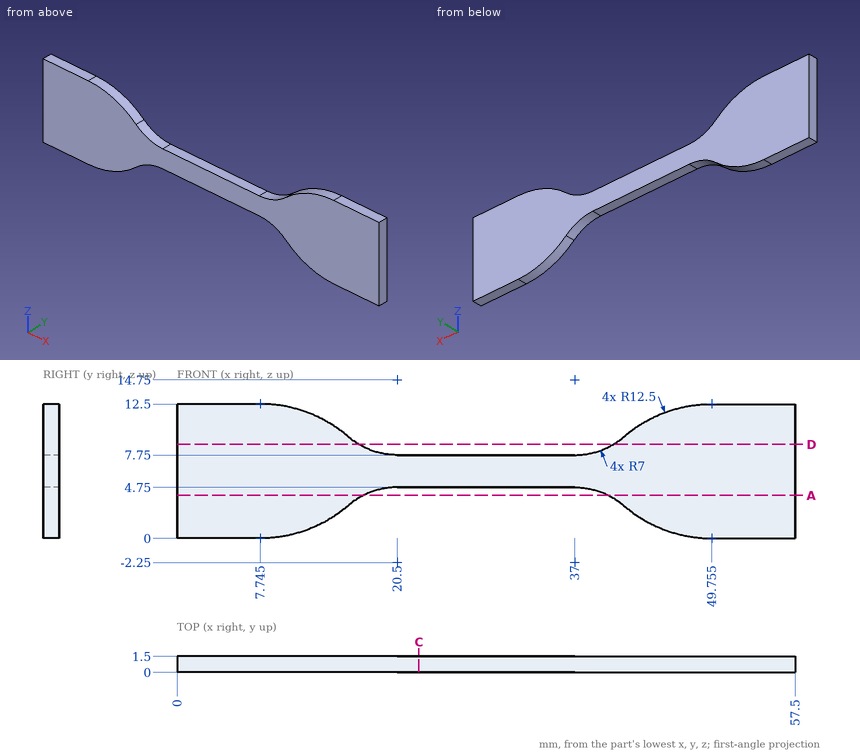
Source: three-view drawing plus pictorial views. Frame: mm from the lowest corner of the part. Give positions to 0.01 mm unless a question says otherwise; leave off trailing zeros. Order: outer loops, then holes, each group sorted by start corner. A loop starts at its lowest first (then second) coordinate and runs counter-clockwise, first axis right, second up. Notation, with made-up numbers: (17.25, 54) - (47.25, 54) arc R16 cw to (47.25, 65) - close; hole circle Ø7 at (1.5, 46.25). An arc over 180 degrees is marked (long way). Answer as a JSON object with one key per item and string values. Group by question number.
Q1. Cut plane C-C, the plane x = 22.5. Output: boundary loops of the cut face in (y, z).
Q2. Line query: probe 1 along Z at (x, y) = (8, 0.75); probe 2 along X at (y, z) = (1, 3.25); probe 3 along X at (y, z) = (1.4, 10.75). Output: solid intervals per line, ascending.
Q3. Cut plane A-A, the plane z = 4. Output: boundary loops of the cut face in (x, y).
Q4. Cut plane D-D, the plane z = 8.75. Output: boundary loops of the cut face in (x, y), then the cut area to 3 significant figures.
Results:
{
 "1": {"outline": "(0, 4.75) - (1.5, 4.75) - (1.5, 7.75) - (0, 7.75) - close"},
 "2": {"probe 1": "0 to 12.5", "probe 2": "0 to 16.17, 41.33 to 57.5", "probe 3": "0 to 14.12, 43.38 to 57.5"},
 "3": {"outline": "(0, 0) - (17.35, 0) - (17.35, 1.5) - (0, 1.5) - close; (40.15, 0) - (57.5, 0) - (57.5, 1.5) - (40.15, 1.5) - close"},
 "4": {"outline": "(0, 0) - (16.89, 0) - (16.89, 1.5) - (0, 1.5) - close; (40.61, 0) - (57.5, 0) - (57.5, 1.5) - (40.61, 1.5) - close", "area": "50.7 mm^2"}
}
